Could you check a few things on this model? Use its own coordinates, in mm. Face numbers are marked on the shaded views. A direction names the side the tool comes from. Coordinates: 2 decimals unless noted, no trailing zeros. Write each loop counter-clockwise with the first axis right and the second up, starting at its lowest first coordinate (ties: lowest second). Pieces come first, ordered by that corner, then holes. Notation, with made-up numbers: M -11.75,55.5 L 2.25,55.5 A24 cw 2.25,71.5 Z; hole C 2,40 d2. An arc over 180 degrees is marked long. Answer as CSV lines item,"result". Start each with the question number.
Item 1: Suppose I cut it at A-A, the plane z = 0. Write out the boundary of the cut face in (x, y) (3 decimals).
Item 2: We'd pull the mould along X, two halves only. Please class the marked faces 3, 4 and 5: +X half, -X half, draft (parallel to the pull), parting line (faces both ways), or undercut.
Item 3: On a 3-axis mill with a long thin cutter (end or side, diameter ignored), from which of +Z, -Z, +X, -X, +Y, -Y can I reach the whole of each face in a straight line? I mean the marked faces 1 and 2. Say none if no direction works.
Item 4: I'm going to push flat-ended pins straight in: P1, Ø1.5, axis at x = -9, z = 6, coming from the -Y side; P2, Ø8, axis at x = 2, y = 21.5, coming from the -Z side (3 decimals); P3, Ø1, axis at x = 3.5, z = -7, coming from the +Y side (3 decimals); P4, Ø3, axis at x = -6.5, y = 19, coming from the +Z side. Where does each tip first touch, or does it pass through?
Item 5: Suppose I cut it at C-C, the plane y = 28. Write out the boundary of the cut face in (x, z) (3 decimals).
Item 6: Suppose I cut it at D-D, the plane z = -8. Write out the boundary of the cut face in (x, y) (3 decimals), and give its area (3 significant figures).
Item 7: If I drill on line 1 along X through (y, z) = (31, 0) (3 decimals); line 2 along X through (y, z) = (11.5, 0) (3 decimals); line 3 along X through (y, z) = (33.5, -5.5), over which ranges is the centre line in solid material (lowest first)? Write a range as [from, to].
Item 8: Suppose I cut it at B-B, the plane x = 0. Write out the boundary of the cut face in (y, z) (3 decimals).
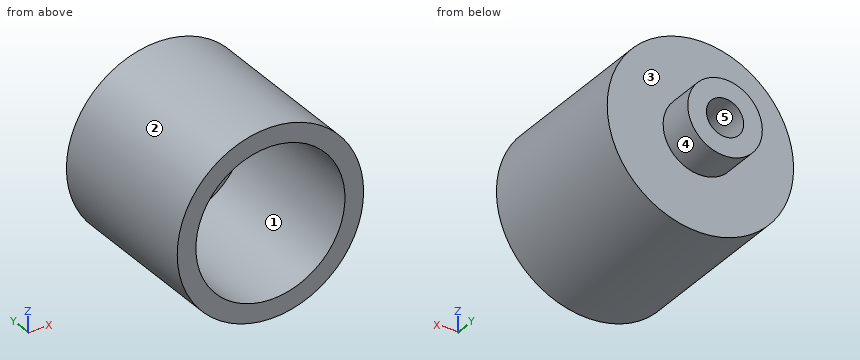
```python
from build123d import *

# Parameters (mm, degrees)
SKETCH1_R           = 15.875
SKETCH1_R_2         = 12.7
BOSS_EXTRUDE1_DEPTH = 25.4
SKETCH2_R           = 15.875
SKETCH2_R_2         = 3.175
BOSS_EXTRUDE2_DEPTH = 3.175
SKETCH3_R           = 6.35
SKETCH3_R_2         = 3.175
BOSS_EXTRUDE3_DEPTH = 6.35


with BuildPart() as part:
    # Sketch1 → Boss-Extrude1 (new body)
    with BuildSketch(Plane(origin=(0, 0, 0), x_dir=(1, 0, 0), z_dir=(0, 1, 0))):
        with Locations(Location((0, 0, 0), (0, 0, 270))):
            Circle(SKETCH1_R)
        with Locations(Location((0, 0, 0), (0, 0, 270))):
            Circle(SKETCH1_R_2, mode=Mode.SUBTRACT)
    extrude(amount=BOSS_EXTRUDE1_DEPTH)

    # Sketch2 → Boss-Extrude2 (add)
    with BuildSketch(Plane(origin=(0, 25.4, 0), x_dir=(1, 0, 0), z_dir=(0, 1, 0))):
        with Locations(Location((0, 0, 0), (0, 0, 270))):
            Circle(SKETCH2_R)
        with Locations(Location((0, 0, 0), (0, 0, 270))):
            Circle(SKETCH2_R_2, mode=Mode.SUBTRACT)
    extrude(amount=BOSS_EXTRUDE2_DEPTH)

    # Sketch3 → Boss-Extrude3 (add)
    with BuildSketch(Plane(origin=(0, 28.575, 0), x_dir=(1, 0, 0), z_dir=(0, 1, 0))):
        with Locations(Location((0, 0, 0), (0, 0, 270))):
            Circle(SKETCH3_R)
        with Locations(Location((0, 0, 0), (0, 0, 270))):
            Circle(SKETCH3_R_2, mode=Mode.SUBTRACT)
    extrude(amount=BOSS_EXTRUDE3_DEPTH)


solid = part.part
```
Ans:
1,outline,"M -15.875,0 L -12.7,0 L -12.7,25.4 L -3.175,25.4 L -3.175,34.925 L -6.35,34.925 L -6.35,28.575 L -15.875,28.575 Z; M 3.175,25.4 L 12.7,25.4 L 12.7,0 L 15.875,0 L 15.875,28.575 L 6.35,28.575 L 6.35,34.925 L 3.175,34.925 Z"
2,face 3,"draft"
2,face 4,"parting line"
2,face 5,"undercut"
3,face 1,"-Y"
3,face 2,"+Y, -Y"
4,P1,"stops at y = 25.4"
4,P2,"stops at z = -15.875"
4,P3,"stops at y = 28.575"
4,P4,"stops at z = 15.07"
5,outline,"C 0,0 d31.75; hole C 0,0 d6.35"
6,outline,"M -13.712,0 L -9.864,0 L -9.864,25.4 L 9.864,25.4 L 9.864,0 L 13.712,0 L 13.712,28.575 L -13.712,28.575 Z"
6,area,"283 mm^2"
7,line 1,"x = [-6.35, -3.175], [3.175, 6.35]"
7,line 2,"x = [-15.875, -12.7], [12.7, 15.875]"
7,line 3,"x = [-3.17, 3.17]"
8,outline,"M 0,-15.875 L 28.575,-15.875 L 28.575,-6.35 L 34.925,-6.35 L 34.925,-3.175 L 25.4,-3.175 L 25.4,-12.7 L 0,-12.7 Z; M 0,12.7 L 25.4,12.7 L 25.4,3.175 L 34.925,3.175 L 34.925,6.35 L 28.575,6.35 L 28.575,15.875 L 0,15.875 Z"
